Design review of the part shown in the three views and the two pictorial views. Dimensions are in mm from the part's minimum x, y and z. Give positions to 0.01 mm unless a question says otherwise; leave off trailing zeros. Loops run counter-clockwise (first coordinate to the right, second up) from the corner with the lowest first, then second, coordinate; pieces in that order, holes last. Notation, with made-up numbers: (53.25, 12.5) - (66.25, 12.5) arc R19 cw to (66.25, 27.5) - close; hole circle Ø11 at (-40, 80). An arc over 180 degrees is marked (long way). Answer in a Markdown table with one row per item.
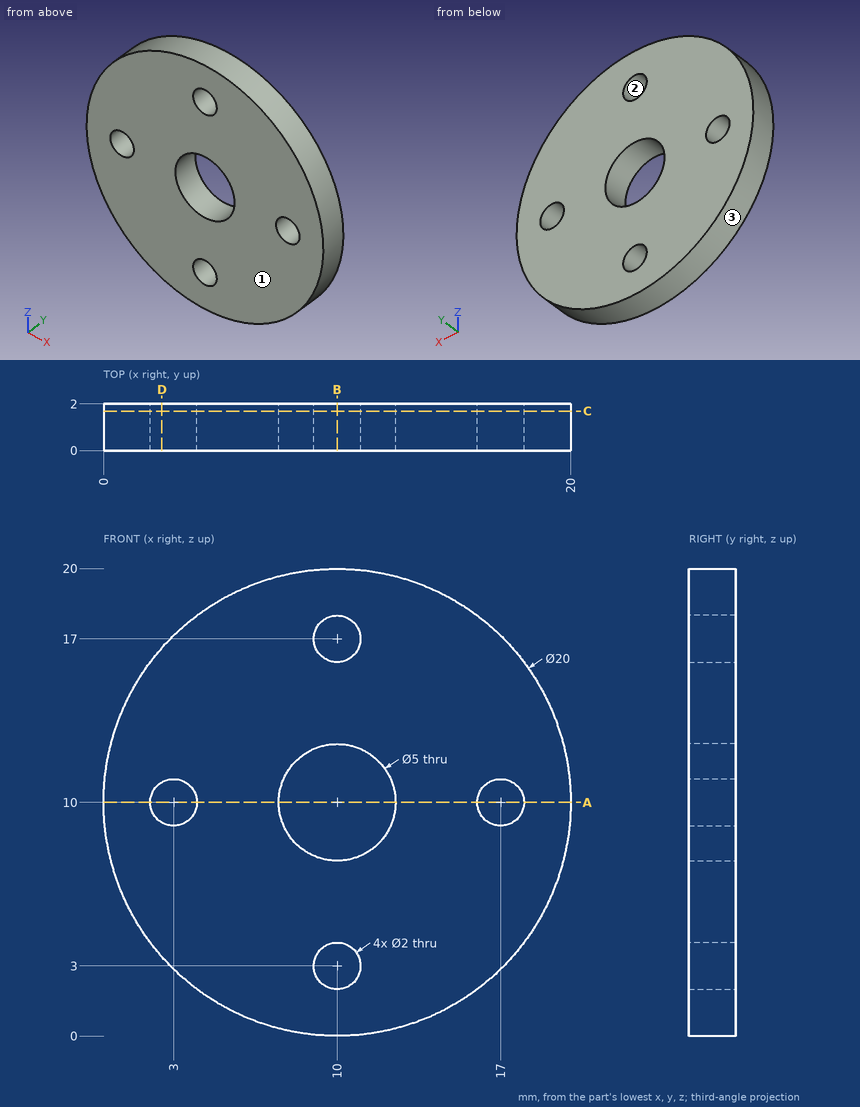
1. Wall thickness on line 1 (X direction, y = 1.6, z = 10); line 2 (Z direction, x = 10.75, y = 1.7); line 3 (Z direction, x = 9.5, y = 0.75): over which ranges is each line inside the solid? List them lowest first. Write a range as [from, to].
Values:
| item | result |
|---|---|
| line 1 | x = [0, 2], [4, 7.5], [12.5, 16], [18, 20] |
| line 2 | z = [0.03, 2.34], [3.66, 7.62], [12.38, 16.34], [17.66, 19.97] |
| line 3 | z = [0.01, 2.13], [3.87, 7.55], [12.45, 16.13], [17.87, 19.99] |
2. We need section B-B, the plane x = 10. Give the boundary of the cut face in (y, z).
Values:
| item | result |
|---|---|
| outline | (0, 0) - (2, 0) - (2, 2) - (0, 2) - close; (0, 4) - (2, 4) - (2, 7.5) - (0, 7.5) - close; (0, 12.5) - (2, 12.5) - (2, 16) - (0, 16) - close; (0, 18) - (2, 18) - (2, 20) - (0, 20) - close |
3. Clearance check with flat-ended pins moving along their axes: pin 1 (2.5 mm diameter, centred on x = 10, z = 3, fed in from -Y); pin 2 (1.8 mm diameter, centred on x = 17, z = 10, fed in from -Y). State where each tip first meets the part, or that it passes through.
Values:
| item | result |
|---|---|
| pin 1 | stops at y = 0 |
| pin 2 | passes through |
4. Mouldability with a two-part tool opening along Z and no side actions: class the marked faces 1, 2 and 3 as released by +Z, released by -Z, zero draft, split by the parting line, or undercut.
Values:
| item | result |
|---|---|
| face 1 | zero draft |
| face 2 | undercut |
| face 3 | split by the parting line |
5. We need section D-D, the plane x = 2.5. Give the boundary of the cut face in (y, z).
Values:
| item | result |
|---|---|
| outline | (0, 3.39) - (2, 3.39) - (2, 9.13) - (0, 9.13) - close; (0, 10.87) - (2, 10.87) - (2, 16.61) - (0, 16.61) - close |
6. We need section A-A, the plane z = 10. Give the boundary of the cut face in (x, y).
Values:
| item | result |
|---|---|
| outline | (0, 0) - (2, 0) - (2, 2) - (0, 2) - close; (4, 0) - (7.5, 0) - (7.5, 2) - (4, 2) - close; (12.5, 0) - (16, 0) - (16, 2) - (12.5, 2) - close; (18, 0) - (20, 0) - (20, 2) - (18, 2) - close |
7. We need section C-C, the plane y = 1.7. Give the boundary of the cut face in (x, z), and give its area (3 significant figures).
Values:
| item | result |
|---|---|
| outline | circle Ø20 at (10, 10); hole circle Ø2 at (3, 10); hole circle Ø5 at (10, 10); hole circle Ø2 at (10, 3); hole circle Ø2 at (10, 17); hole circle Ø2 at (17, 10) |
| area | 282 mm^2 |
